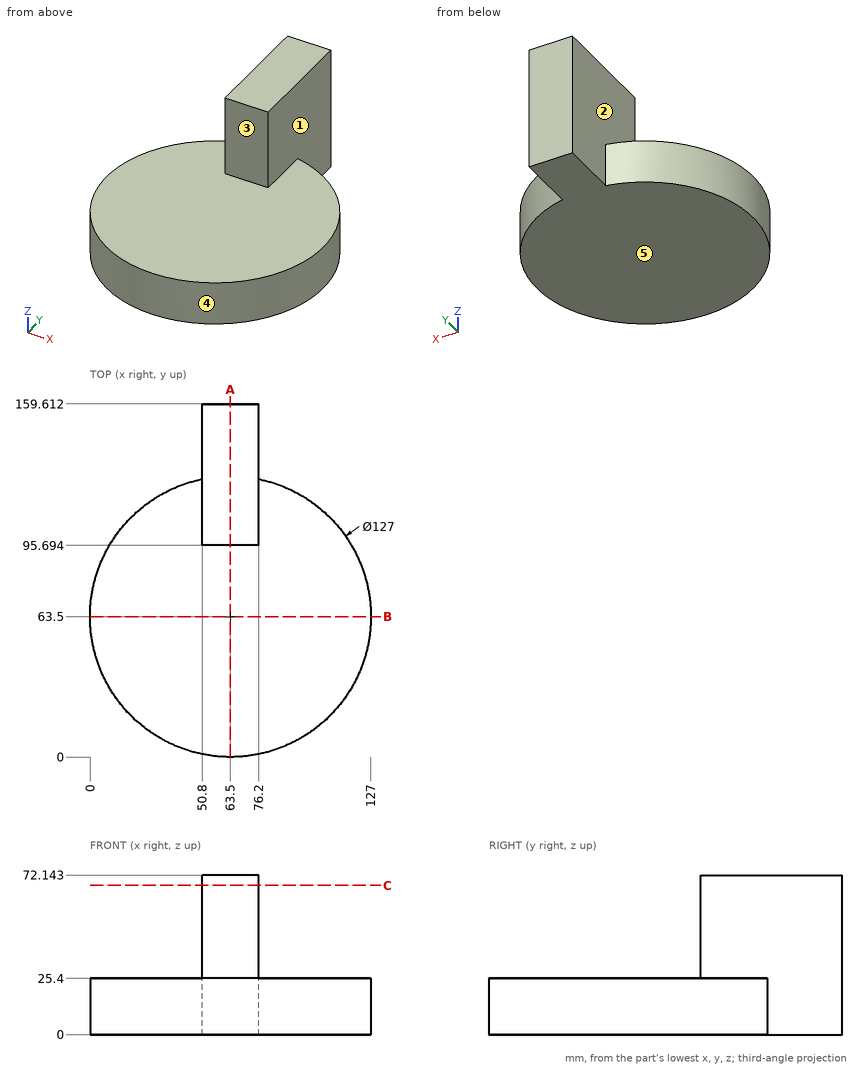
Design review of the part shown in the three views and the two pictorial views. Dimensions are in mm from the part's minimum x, y and z. A direction names the side the tool comes from. Give positions to 0.01 mm unless a question says otherwise; leave off trailing zeros. Loops run counter-clockwise (first coordinate to the right, second up) from the corner with the lowest first, then second, coordinate; pieces in that order, holes last. Notation, with made-up numbers: (-6.75, 4.25) -> (8.25, 4.25) arc R20 ccw to (8.25, 15.25) -> close; hole circle Ø8 at (73.25, -19). An arc over 180 degrees is marked (long way). Put each result on its own line as item: value. Start each with the question number.
1. We need section C-C on z = 67.5. State the section outline as (x, y) points, then the cut area to 3 significant figures.
2. We need section A-A on x = 63.5. State the section outline as (y, z) points, then the cut area to 3 significant figures.
3. We need section B-B on y = 63.5. State the section outline as (x, z) points.
4. Wall thickness on probe 1 along X at (y, z) = (125, 43); probe 2 along Z at (x, y) = (49.5, 75); probe 3 along Y at (x, z) = (74, 51.5): over which ranges is each line inside the solid? List them lowest first.
5. For the marked faces 1, 2, 3, 4 and 5, list the 3-axis set-ups (+Z, -Z, +X, -X, +Y, -Y) from which the entire face can be reached by the end or side of a thin tool; tool diameter is ignored.
6. Clearance check with flat-ended pins moving along their axes: P1, Ø7.5, axis at x = 58, z = 51, coming from the -Y side; P2, Ø4, axis at x = 79, y = 65, coming from the -Z side; P3, Ø12, axis at x = 72.5, z = 14.5, coming from the -Y side; P4, Ø1, axis at y = 95, z = 25.5, coming from the +X side. State where each tip first meets the part, or that it passes through.
Determined:
1. outline: (50.8, 95.69) -> (76.2, 95.69) -> (76.2, 159.61) -> (50.8, 159.61) -> close
1. area: 1,620 mm^2
2. outline: (0, 0) -> (159.61, 0) -> (159.61, 72.14) -> (95.69, 72.14) -> (95.69, 25.4) -> (0, 25.4) -> close
2. area: 7,040 mm^2
3. outline: (0, 0) -> (127, 0) -> (127, 25.4) -> (0, 25.4) -> close
4. probe 1: 50.8 to 76.2
4. probe 2: 0 to 25.4
4. probe 3: 95.69 to 159.61
5. face 1: +Z, +X, +Y
5. face 2: +Z, -X, +Y
5. face 3: +Z, +X, -X, -Y
5. face 4: +Z, -Z
5. face 5: -Z, +X, -X, +Y, -Y
6. P1: y = 95.69
6. P2: z = 0
6. P3: y = 0.07
6. P4: x = 118.91
